from build123d import *

# Parameters (mm, degrees)
SKETCH1_W           = 70
SKETCH1_H           = 83.94
BOSS_EXTRUDE1_DEPTH = 8
BOSS_EXTRUDE2_START = -10
SKETCH3_R           = 5.1
SKETCH3_R_2         = 3.1
BOSS_EXTRUDE2_DEPTH = 5
CUT_EXTRUDE1_DEPTH  = 63
BOSS_EXTRUDE3_DEPTH = 5
SKETCH6_R           = 2
BOSS_EXTRUDE4_DEPTH = 3.8
BOSS_EXTRUDE4_TAPER = 14
FILLET1_R           = 1


with BuildPart() as part:
    # Sketch1 → Boss-Extrude1 (new body)
    with BuildSketch(Plane(origin=(0, 0, 0), x_dir=(1, 0, 0), z_dir=(0, 1, 0))):
        Rectangle(SKETCH1_W, SKETCH1_H)
    extrude(amount=BOSS_EXTRUDE1_DEPTH)

    # Sketch3 → Boss-Extrude2 (add)
    # profile 1 of 2: a face of its own
    with BuildSketch(Plane(origin=(0, 0, -41.97), x_dir=(-1, 0, 0), z_dir=(0, 0, -1)).offset(BOSS_EXTRUDE2_START)):
        with Locations((-30, -4.1)):
            Circle(SKETCH3_R)
        with Locations((-30, -4.1)):
            Circle(SKETCH3_R_2, mode=Mode.SUBTRACT)
    # profile 2 of 2: a face of its own
    with BuildSketch(Plane(origin=(0, 0, -41.97), x_dir=(-1, 0, 0), z_dir=(0, 0, -1)).offset(BOSS_EXTRUDE2_START)):
        with Locations((30, -4.1)):
            Circle(SKETCH3_R)
        with Locations((30, -4.1)):
            Circle(SKETCH3_R_2, mode=Mode.SUBTRACT)
    boss_extrude2 = extrude(amount=-BOSS_EXTRUDE2_DEPTH)

    # Mirror1: Boss-Extrude2 across plane
    add(boss_extrude2.mirror(Plane.XY.offset(-13.22)))

    # Sketch4 → Cut-Extrude1 (cut)
    with BuildSketch(Plane.XY.offset(5.53)):
        Polygon((30, -4.1), (40, -9.873502692), (20, -9.873502692), align=None)
        Polygon((-40, -9.873502692), (-20, -9.873502692), (-30, -4.1), align=None)
    extrude(amount=-CUT_EXTRUDE1_DEPTH, mode=Mode.SUBTRACT)


with BuildPart() as body_2:
    # Sketch5 → Boss-Extrude3 (new body)
    with BuildSketch(Plane.XY.offset(41.97)):
        with BuildLine():
            Line((35, 8), (35.5, 8))
            ThreePointArc((35.5, 8), (41.352973318, 11.544924524), (41.783244941, 4.715674721))
            Line((41.783244941, 4.715674721), (35, 0))
            Line((35, 0), (35, 8))
        make_face()
    extrude(amount=-BOSS_EXTRUDE3_DEPTH)

    # Sketch6 → Boss-Extrude4 (add)
    with BuildSketch(Plane(origin=(0, 0, 36.97), x_dir=(-1, 0, 0), z_dir=(0, 0, -1))):
        with Locations((-39.5, 8)):
            Circle(SKETCH6_R)
    extrude(amount=BOSS_EXTRUDE4_DEPTH, taper=BOSS_EXTRUDE4_TAPER)

    # Fillet1
    fillet1_edges = [body_2.edges().sort_by_distance(p)[0] for p in [
        (40.552553589, 8, 33.17),
    ]]
    fillet(fillet1_edges, radius=FILLET1_R)


with BuildPart() as body_3:
    # Mirror2: mirrored copy
    add(body_2.part.mirror(Plane(origin=(0, 4, 0), x_dir=(0, 0, 1), z_dir=(0, -1, 0))))


with BuildPart() as body_3_2:
    # Mirror3: mirrored copy
    add(body_3.part.mirror(Plane.XY))


with BuildPart() as body_4:
    # Mirror4: mirrored copy
    add(body_3.part.mirror(Plane.ZY))


with BuildPart() as body_5:
    # Mirror4 2: mirrored copy
    add(body_3_2.part.mirror(Plane.ZY))

    # Combine1: union part, body 4, body 3, body 3 2
    add(part.part)
    add(body_4.part)
    add(body_3.part)
    add(body_3_2.part)


solid = body_5.part
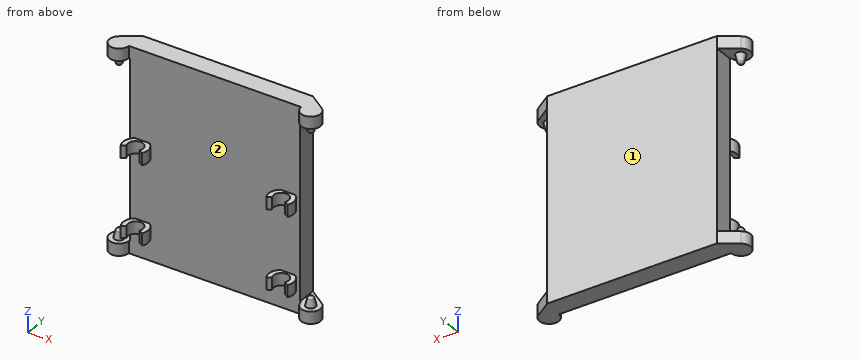
The listing builds one solid part. Answer for the finished solid, in the listing's coordinates (mm). Face numbers are marked on the shaded views. Round coordinates to 2 decimals unless told otherwise and drop trailing zeros. Order: outer loops, then holes, each group sorted by start corner. A loop starts at its lowest first (then second) coordinate and runs counter-clockwise, first axis right, second up. Notation, with made-up numbers: M 13.25,82.25 L 60.25,82.25 A10 cw 60.25,94.25 Z; hole C 56.5,28 d10. An arc over 180 degrees is marked long. Answer in a Markdown table with one row per item. Add a question column.
1) The part is cut by section D-D on x = 16. Determine the outline of the cut face in (y, z).
2) The part is cut by section C-C on y = 4.5. Determine the outline of the cut face in (x, z).
3) Consider line 1 along X through (y, z) = (-4.1, 4.2); line 2 along Z through (x, y) = (40.5, -2.5); line 3 along X through (y, z) = (1.75, 35.5). Determine where each line is inside the solid, lowest interval first. Write a range as from..to.
4) Flat-ended cylindrical pins translate along their axes: pin 1 Ø3 at (y, z) = (5.5, -29.5) entering from +X; pin 2 Ø3 at (y, z) = (0, -29) entering from -X; pin 3 Ø2 at (x, y) = (-29.5, -4) entering from -Z; pin 4 Ø2 at (x, y) = (32, -2) entering from +Z. Find the tip coordinate at first contact, or state that the pin passes through.
5) Determine the mould class of the marked faces 1 and 2 for opening direction X: pulls with the +X half, pulls with the -X half, needs draft (parallel to the pull), parting line crosses it, or undercut.
6) The part is cut by section B-B on z = -28. Determine the outline of the cut face in (x, y).
7) The part is cut by section A-A on x = -30. Determine the outline of the cut face in (y, z).
Findings below:
| question | item | result |
|---|---|---|
| 1 | outline | M 0,-41.97 L 8,-41.97 L 8,41.97 L 0,41.97 Z |
| 2 | outline | M -40.03,-41.97 L 40.03,-41.97 L 40.03,-36.97 L 35,-36.97 L 35,36.97 L 40.03,36.97 L 40.03,41.97 L -40.03,41.97 L -40.03,36.97 L -35,36.97 L -35,-36.97 L -40.03,-36.97 Z |
| 3 | line 1 | x = -35.1..-33.1, -26.9..-24.9, 24.9..26.9, 33.1..35.1 |
| 3 | line 2 | z = -41.97..-36.97, 36.97..41.97 |
| 3 | line 3 | x = -35..35 |
| 4 | pin 1 | stops at x = 35 |
| 4 | pin 2 | stops at x = -35 |
| 4 | pin 3 | passes through |
| 4 | pin 4 | stops at z = 5.53 |
| 5 | face 1 | needs draft |
| 5 | face 2 | undercut |
| 6 | outline | M -35,0 L -33.03,0 A5.1 ccw -34.42,-6.65 L -32.68,-5.65 A3.1 cw long -27.32,-5.65 L -25.58,-6.65 A5.1 ccw -26.97,0 L 26.97,0 A5.1 ccw 25.58,-6.65 L 27.32,-5.65 A3.1 cw long 32.68,-5.65 L 34.42,-6.65 A5.1 ccw 33.03,0 L 35,0 L 35,8 L -35,8 Z |
| 7 | outline | M -1,-31.97 L 0,-31.97 L 0,-41.97 L 8,-41.97 L 8,41.97 L 0,41.97 L 0,5.53 L -1,5.53 L -1,0.53 L 0,0.53 L 0,-26.97 L -1,-26.97 Z |
